Build history of the part. All positions in model axes, mm. A direction names the side the tool comes from. Round coordinates to 2 decimals unless told otherwise and drop trailing zeros. Loops run counter-clockwise (first coordinate to the right, second up) from the corner with the lowest first, then second, coordinate; pieces in that order, holes last. Notation, with made-up numbers: (-14.5, -38) -> (36.5, -38) arc R11 ccw to (36.5, -27) -> close; hole circle Ø9 at (-30.75, 26). An arc over 180 degrees is marked (long way). Put each result on its own line as item: value. Start each with the question number.
Item 1: Tool access for faces 1 (the flat face through (2.4, 1.2, 6.1)), 2 (the flat face through (0, 0, 9.5)): list every direction of +Z, -Z, +X, -X, +Y, -Y with a clear straight run to the whole face (end or side of a thin tool).
Item 2: Flat gauge pins, fed straight in: pin 1 Ø4 at (x, y) = (3.5, 7.5) entering from -Z; pin 2 Ø1 at (y, z) = (1.5, 2) entering from +X; pin 3 Ø1.5 at (y, z) = (3.5, 8) entering from +X. Where does each tip first touch, or does it go through?
Item 3: Cut at D-D, the plane x = 4. List the corners of the cut face in (y, z), plus the area to 3 significant figures.
Item 4: Drill centre lines: probe 1 along Z at (x, y) = (-8.5, 0); probe 2 along Z at (x, y) = (1, -4.75); probe 3 along Y at (x, z) = (0, 7.25). Where is each one in solid material? Low to high. Write a range as [from, to].
Item 5: Cut at A-A, the plane y = 0. List the corners of the cut face in (x, z).
Item 6: Cut at C-C, the plane z = 1.25. List the corners of the cut face in (x, y).
```python
from build123d import *

# Parameters (mm, degrees)
F0_R       = 2.35
F1_DEPTH   = 7.5
F2_R       = 10
F3_DEPTH   = 2
F4_R       = 5.65
F1_FACE1_R = 2.35
F5_DEPTH   = 1.4


with BuildPart() as f1:
    # F0 (on Top) → F1 (new body)
    with BuildSketch(Plane.XY):
        Circle(F0_R)
    extrude(amount=F1_DEPTH)

    # F2 (on face) → F3 (join)
    with BuildSketch(Plane.XY.offset(7.5)):
        Circle(F2_R)
    extrude(amount=F3_DEPTH)

    # F4 (on face) + F1_face1 (on face) → F5 (join)
    with BuildSketch(Plane(origin=(0, 0, 7.5), x_dir=(1, 0, 0), z_dir=(0, 0, -1))):
        Circle(F4_R)
    with BuildSketch(Plane(origin=(0, 0, 0), x_dir=(1, 0, 0), z_dir=(0, 0, -1))):
        Circle(F1_FACE1_R)
    extrude(amount=F5_DEPTH)


solid = f1.part
```
Reply:
1. face 1: -Z
1. face 2: +Z, +X, -X, +Y, -Y
2. pin 1: stops at z = 7.5
2. pin 2: stops at x = 2.13
2. pin 3: stops at x = 9.61
3. outline: (-9.17, 7.5) -> (-3.99, 7.5) -> (-3.99, 6.1) -> (3.99, 6.1) -> (3.99, 7.5) -> (9.17, 7.5) -> (9.17, 9.5) -> (-9.17, 9.5) -> close
3. area: 47.8 mm^2
4. probe 1: z = [7.5, 9.5]
4. probe 2: z = [6.1, 9.5]
4. probe 3: y = [-5.65, 5.65]
5. outline: (-10, 7.5) -> (-5.65, 7.5) -> (-5.65, 6.1) -> (-2.35, 6.1) -> (-2.35, -1.4) -> (2.35, -1.4) -> (2.35, 6.1) -> (5.65, 6.1) -> (5.65, 7.5) -> (10, 7.5) -> (10, 9.5) -> (-10, 9.5) -> close
6. outline: circle Ø4.7 at (0, 0)
